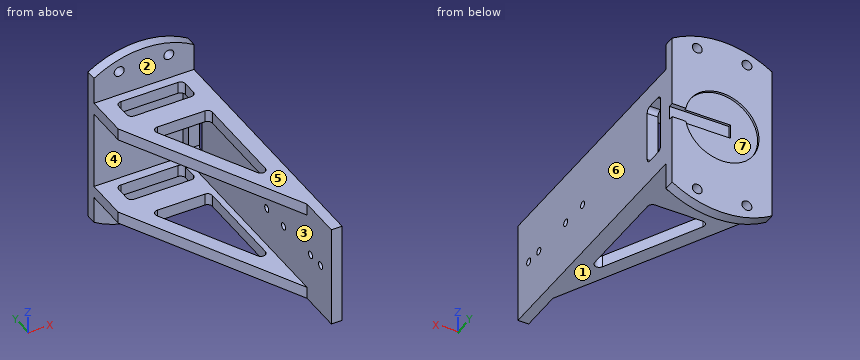
```python
from build123d import *

# Parameters (mm, degrees)
SKETCH1_R           = 2.1
BOSS_EXTRUDE1_DEPTH = 4.5
SKETCH2_R           = 15.5
CUT_EXTRUDE1_DEPTH  = 1
SKETCH3_W           = 25
SKETCH3_H           = 6
CUT_EXTRUDE2_DEPTH  = 2
BOSS_EXTRUDE2_DEPTH = 110
CUT_EXTRUDE3_DEPTH  = 128.284130983
CUT_EXTRUDE4_REACH  = 126.036
SKETCH6_R           = 1.5
CUT_EXTRUDE5_REACH  = 124.586
CUT_EXTRUDE6_DEPTH  = 110


with BuildPart() as part:
    # Sketch1 → Boss-Extrude1 (new body)
    with BuildSketch(Plane(origin=(0, 0, 0), x_dir=(1, 0, 0), z_dir=(0, 1, 0))):
        with BuildLine():
            Line((-21, 32.86335345), (-21, -32.86335345))
            ThreePointArc((-21, -32.86335345), (0, -39), (21, -32.86335345))
            Line((21, -32.86335345), (21, 32.86335345))
            ThreePointArc((21, 32.86335345), (0, 39), (-21, 32.86335345))
        make_face()
        with Locations(Location((10.42932356, 32.098157425, 0), (0, 0, 270))):
            Circle(SKETCH1_R, mode=Mode.SUBTRACT)
        with Locations(Location((-10.42932356, 32.098157425, 0), (0, 0, 270))):
            Circle(SKETCH1_R, mode=Mode.SUBTRACT)
        with Locations(Location((10.42932356, -32.098157425, 0), (0, 0, 270))):
            Circle(SKETCH1_R, mode=Mode.SUBTRACT)
        with Locations(Location((-10.42932356, -32.098157425, 0), (0, 0, 270))):
            Circle(SKETCH1_R, mode=Mode.SUBTRACT)
    extrude(amount=BOSS_EXTRUDE1_DEPTH)

    # Sketch2 → Cut-Extrude1 (cut)
    with BuildSketch(Plane(origin=(0, 4.5, 0), x_dir=(1, 0, 0), z_dir=(0, 1, 0))):
        with Locations(Location((0, 0, 0), (0, 0, 270))):
            Circle(SKETCH2_R)
    extrude(amount=-CUT_EXTRUDE1_DEPTH, mode=Mode.SUBTRACT)

    # Sketch3 → Cut-Extrude2 (cut)
    with BuildSketch(Plane(origin=(0, 4.5, 0), x_dir=(1, 0, 0), z_dir=(0, 1, 0))):
        with Locations((8.5, 0)):
            Rectangle(SKETCH3_W, SKETCH3_H)
    extrude(amount=-CUT_EXTRUDE2_DEPTH, mode=Mode.SUBTRACT)

    # Sketch4 → Boss-Extrude2 (add)
    with BuildSketch(Plane.XZ):
        Polygon((21, 21.5), (-21, 21.5), (-21, 16.5), (-16.5, 16.5), (16.5, 16.5), (16.5, -16.5), (-16.5, -16.5), (-21, -16.5), (-21, -21.5), (21, -21.5), align=None)
    extrude(amount=BOSS_EXTRUDE2_DEPTH)

    # Sketch5 → Cut-Extrude3 (cut, through all)
    with BuildSketch(Plane.XY.offset(21.5)):
        Polygon((-21, -18), (16.5, -110), (16.5, -92), align=None)
    extrude(amount=-CUT_EXTRUDE3_DEPTH, mode=Mode.SUBTRACT)


with BuildPart() as cut_extrude3_kept_piece:
    # of the separate pieces the step leaves, the one the design keeps (cut_extrude3_pieces_kept)
    add(part.part.solids().sort_by_distance((21, 0, -32.86335345))[0])

    # Sketch6 → Cut-Extrude4 (cut, up to next)
    with BuildSketch(Plane(origin=(21, 0, 0), x_dir=(0, 0, -1), z_dir=(1, 0, 0)), mode=Mode.PRIVATE) as cut_extrude4_sk1:
        with Locations((0, -102)):
            Circle(SKETCH6_R)
    cut_extrude4_tool1 = extrude(cut_extrude4_sk1.sketch, amount=-CUT_EXTRUDE4_REACH, mode=Mode.PRIVATE) & cut_extrude3_kept_piece.part
    # Sketch6 → Cut-Extrude4 (cut, up to next)
    with BuildSketch(Plane(origin=(21, 0, 0), x_dir=(0, 0, -1), z_dir=(1, 0, 0)), mode=Mode.PRIVATE) as cut_extrude4_sk2:
        with Locations((0, -94.5)):
            Circle(SKETCH6_R)
    cut_extrude4_tool2 = extrude(cut_extrude4_sk2.sketch, amount=-CUT_EXTRUDE4_REACH, mode=Mode.PRIVATE) & cut_extrude3_kept_piece.part
    # Sketch6 → Cut-Extrude4 (cut, up to next)
    with BuildSketch(Plane(origin=(21, 0, 0), x_dir=(0, 0, -1), z_dir=(1, 0, 0)), mode=Mode.PRIVATE) as cut_extrude4_sk3:
        with Locations((0, -74.5)):
            Circle(SKETCH6_R)
    cut_extrude4_tool3 = extrude(cut_extrude4_sk3.sketch, amount=-CUT_EXTRUDE4_REACH, mode=Mode.PRIVATE) & cut_extrude3_kept_piece.part
    # Sketch6 → Cut-Extrude4 (cut, up to next)
    with BuildSketch(Plane(origin=(21, 0, 0), x_dir=(0, 0, -1), z_dir=(1, 0, 0)), mode=Mode.PRIVATE) as cut_extrude4_sk4:
        with Locations((0, -62)):
            Circle(SKETCH6_R)
    cut_extrude4_tool4 = extrude(cut_extrude4_sk4.sketch, amount=-CUT_EXTRUDE4_REACH, mode=Mode.PRIVATE) & cut_extrude3_kept_piece.part
    add(cut_extrude4_tool1.solids().sort_by_distance((21, -102, 0))[0], mode=Mode.SUBTRACT)
    add(cut_extrude4_tool2.solids().sort_by_distance((21, -94.5, 0))[0], mode=Mode.SUBTRACT)
    add(cut_extrude4_tool3.solids().sort_by_distance((21, -74.5, 0))[0], mode=Mode.SUBTRACT)
    add(cut_extrude4_tool4.solids().sort_by_distance((21, -62, 0))[0], mode=Mode.SUBTRACT)

    # Sketch7 → Cut-Extrude5 (cut, up to next)
    with BuildSketch(Plane.ZY.offset(-16.5), mode=Mode.PRIVATE) as cut_extrude5_sk1:
        with BuildLine():
            Line((-10.5, -4), (10.5, -4))
            ThreePointArc((10.5, -4), (11.914213562, -4.585786438), (12.5, -6))
            Line((12.5, -6), (12.5, -12))
            ThreePointArc((12.5, -12), (11.914213562, -13.414213562), (10.5, -14))
            Line((10.5, -14), (-10.5, -14))
            ThreePointArc((-10.5, -14), (-11.914213562, -13.414213562), (-12.5, -12))
            Line((-12.5, -12), (-12.5, -6))
            ThreePointArc((-12.5, -6), (-11.914213562, -4.585786438), (-10.5, -4))
        make_face()
    cut_extrude5_tool1 = extrude(cut_extrude5_sk1.sketch, amount=-CUT_EXTRUDE5_REACH, mode=Mode.PRIVATE) & cut_extrude3_kept_piece.part
    add(cut_extrude5_tool1.solids().sort_by_distance((16.5, -9, 0))[0], mode=Mode.SUBTRACT)

    # Sketch8 → Cut-Extrude6 (cut)
    with BuildSketch(Plane.XY.offset(21.5)):
        with BuildLine():
            Line((-7.977370013, -24), (12, -24))
            ThreePointArc((12, -24), (13.414213562, -24.585786438), (14, -26))
            Line((14, -26), (14, -65.422010158))
            ThreePointArc((14, -65.422010158), (12.46475074, -67.36726252), (10.21599325, -66.326067633))
            Line((10.21599325, -66.326067633), (-9.761376762, -26.904057474))
            ThreePointArc((-9.761376762, -26.904057474), (-9.681499548, -24.953127264), (-7.977370013, -24))
        make_face()
        with BuildLine():
            Line((-12, -14), (12, -14))
            ThreePointArc((12, -14), (13.414213562, -13.414213562), (14, -12))
            Line((14, -12), (14, -6))
            ThreePointArc((14, -6), (13.414213562, -4.585786438), (12, -4))
            Line((12, -4), (-12, -4))
            ThreePointArc((-12, -4), (-13.414213562, -4.585786438), (-14, -6))
            Line((-14, -6), (-14, -12))
            ThreePointArc((-14, -12), (-13.414213562, -13.414213562), (-12, -14))
        make_face()
    extrude(amount=-CUT_EXTRUDE6_DEPTH, mode=Mode.SUBTRACT)


solid = cut_extrude3_kept_piece.part
```
Geometry check sheet. Reference: the model listing, model coordinates, mm. Face numbers are marked on the shaded views. A direction names the side the tool comes from. Coordinates: 2 decimals unless noted, no trailing zeros. Order: outer loops, then holes, each group sorted by start corner. A loop starts at its lowest first (then second) coordinate and runs counter-clockwise, first axis right, second up. Notation, with made-up numbers: (7, -37) - (18, -37) arc R28 cw to (18, -13) - close; hole circle Ø10 at (49, 72.5). An arc over 180 degrees is marked (long way). Answer in a Markdown table with one row per item. Add a question column.
1. Gauge pin test, flat ends, axial feed: pin 1 Ø2 at (x, z) = (8.5, -30) entering from -Y; pin 2 Ø12 at (x, y) = (1, -63.5) entering from +Z; pin 3 Ø2 at (y, z) = (-37.5, -4) entering from -X; pin 4 Ø4 at (x, z) = (-10.43, 32.1) entering from -Y. Record the tip position at first contact, or that the pin passes through.
2. Section check A-A (y = -94.5). Enter the section's corners in (x, z).
3. Section check D-D (y = -62). Enter the section's corners in (x, z).
4. Section check C-C (z = 8.5). Enter the section's corners in (x, y).
5. Draft check along Z on the marked faces 1, 2 and 3. Enter one of: +Z half, -Z half, draft (parallel to the pull), parting line (faces both ways), or undercut.
6. Access from +Z, -Z, +X, -X, +Y, -Y to the whole of each face (thin tool, end or side, straight path). Record for the marked faces 4, 5, 6 and 7.
7. Section check B-B (z = 0). Give the number of separate pieces and of enclosed holes in the cut face, plus the area to 4 significant figures.
8. Material ranges on L1, parallel to Z at x = -1, y = -21.5; L2, parallel to Y at x = 18, z = 0; L3, parallel to Z at x = 18.55, y = -102, recorded low to high. Write a range as [from, to].
Data:
| question | item | result |
|---|---|---|
| 1 | pin 1 | stops at y = 0 |
| 1 | pin 2 | stops at z = 21.5 |
| 1 | pin 3 | stops at x = 16.5 |
| 1 | pin 4 | passes through |
| 2 | outline | (16.5, -21.5) - (21, -21.5) - (21, -1.5) - (16.5, -1.5) - close; (16.5, 1.5) - (21, 1.5) - (21, 21.5) - (16.5, 21.5) - close |
| 3 | outline | (1.3, -21.5) - (8.02, -21.5) - (8.02, -16.5) - (1.3, -16.5) - close; (1.3, 16.5) - (8.02, 16.5) - (8.02, 21.5) - (1.3, 21.5) - close; (14, -21.5) - (21, -21.5) - (21, -1.5) - (16.5, -1.5) - (16.5, -16.5) - (14, -16.5) - close; (14, 16.5) - (16.5, 16.5) - (16.5, 1.5) - (21, 1.5) - (21, 21.5) - (14, 21.5) - close |
| 4 | outline | (-21, 0) - (16.5, 0) - (16.5, -4) - (21, -4) - (21, 4.5) - (12.96, 4.5) - (12.96, 3.5) - (-12.96, 3.5) - (-12.96, 4.5) - (-21, 4.5) - close; (16.5, -110) - (21, -110) - (21, -14) - (16.5, -14) - close |
| 5 | face 1 | -Z half |
| 5 | face 2 | draft |
| 5 | face 3 | undercut |
| 6 | face 4 | -X, -Y |
| 6 | face 5 | +Z, +X, -X, -Y |
| 6 | face 6 | +Z, -Z, +X, +Y, -Y |
| 6 | face 7 | +Y |
| 7 | separate pieces | 6 |
| 7 | enclosed holes | 0 |
| 7 | area | 523.5 mm² |
| 8 | L1 | z = [-21.5, -16.5], [16.5, 21.5] |
| 8 | L2 | y = [-110, -103.5], [-100.5, -96], [-93, -76], [-73, -63.5], [-60.5, -14], [-4, 2.5] |
| 8 | L3 | z = [-21.5, -1.5], [1.5, 21.5] |
